Autodesk Inventor part; units mm, degrees
ref_plane "YZ Plane" through (0, 0, 0) normal (1, 0, 0) x (0, 1, 0)
ref_plane "XZ Plane" through (0, 0, 0) normal (0, 1, 0) x (-1, 0, 0)
ref_plane "XY Plane" through (0, 0, 0) normal (0, 0, 1) x (1, 0, 0)
sketch "スケッチ1" plane through (0, 0, 0) normal (0, 0, 1) x (1, 0, 0)
  circle A0 centre (0, 5.8) radius 2.6
  circle A1 centre (0, 13.4) radius 2.6
  line L0 (-3.8, 0) -> (3.8, 0)
  line L1 (3.8, 0) -> (3.8, 17.6)
  line L2 (3.8, 17.6) -> (-3.8, 17.6)
  line L3 (-3.8, 17.6) -> (-3.8, 0)
  line L4 (-11.5586, 9.6) -> (11.5586, 9.6) construction
  point P0 (0, 0)
  point P1 (0, 0)
  point P2 (0, 9.6)
  dimension "LED_DIA" = 5.2
  dimension "d1" = 7.6
  dimension "LED_PITCH" = 7.6
  dimension "TOP_MARGIN" = 4.2
  dimension "BOTTOM_MARGIN" = 5.8
extrude "スペーサ" add sketch "スケッチ1" along normal blind 5
sketch "スケッチ2" plane through (0, 0, 0) normal (0, 0, -1) x (-1, 0, 0)
  line L0 (3.8, 17.6) -> (3.8, 0)
  line L1 (-3.8, 0) -> (-3.8, 17.6)
  line L2 (3.8, 0) -> (-3.8, 0)
  line L3 (-3.8, 0) -> (-3.8, 2)
  line L4 (-3.8, 2) -> (3.8, 2)
  line L5 (3.8, 2) -> (3.8, 0)
  line L6 (3.8, 10.2) -> (-3.8, 10.2)
  line L7 (-3.8, 10.2) -> (-3.8, 9)
  line L8 (-3.8, 9) -> (3.8, 9)
  line L9 (3.8, 9) -> (3.8, 10.2)
  circle A0 centre (0, 5.8) radius 2.9 construction
  circle A1 centre (0, 13.4) radius 2.9 construction
  circle A2 centre (0, 5.8) radius 2.6 construction
  circle A3 centre (0, 13.4) radius 2.6 construction
  line L10 (6.2058, 13.4) -> (-6.2058, 13.4) construction
  line L11 (-6.2058, 5.8) -> (6.2058, 5.8) construction
  line L12 (6.2058, 9.6) -> (-6.2058, 9.6) construction
  point P0 (0, 0)
  point P1 (3.8, 9.6)
  point P2 (-3.8, 9)
  point P3 (3.8, 9)
  point P4 (3.8, 10.2)
  point P5 (-3.8, 10.2)
  dimension "d8" = 5.8
  dimension "d9" = 2
  dimension "d10" = 1.2
extrude "押し出し2" add sketch "スケッチ2" along normal blind 3 contours L0 L2 L1 L4
extrude "押し出し5" add sketch "スケッチ2" along normal blind 2 contours L0 L8 L1 L6
chamfer "面取り1" distance 0.6 angle 45 1 edges at (-2.6, 13.4, 5)
sketch "スケッチ4" plane through (-3.8, 0, 5) normal (0, -1, 0) x (1, 0, 0)
  line L0 (4.55, -5) -> (3.05, -5)
  line L1 (3.05, -5) -> (2.3, -3.701)
  line L2 (2.3, -3.701) -> (3.05, -2.4019)
  line L3 (3.05, -2.4019) -> (4.55, -2.4019)
  line L4 (4.55, -2.4019) -> (5.3, -3.701)
  line L5 (5.3, -3.701) -> (4.55, -5)
  line L6 (0, 0) -> (7.6, 0)
  point P0 (3.8, -5)
  point P1 (3.8, -3.701)
  dimension "d19" = 3
extrude "足" add sketch "スケッチ4" along normal blind 3
sketch "スケッチ5" plane through (0, 0, 5) normal (0, 0, 1) x (1, 0, 0)
  line L0 (-0.1, 5.8) -> (0.1, 5.8)
  line L1 (0.1, 5.8) -> (0.1, 17.6)
  line L2 (0.1, 17.6) -> (-0.1, 17.6)
  line L3 (-0.1, 17.6) -> (-0.1, 5.8)
  line L4 (-3.8, 0) -> (3.8, 0)
  line L5 (3.8, 17.6) -> (-3.8, 17.6)
  point P0 (0, 0)
  point P1 (0, 5.8)
  point P2 (0, 0)
  dimension "d24" = 0.2
extrude "押し出し6" cut sketch "スケッチ5" against normal blind 0.2
properties part number "LED-Spacer1"
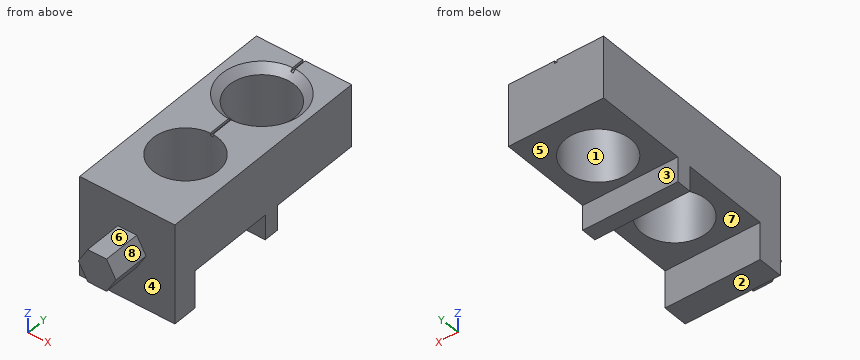
CAD build for the part. Positions are in the model's coordinates, mm. Face numbers are marked on the shaded views. A direction names the side the tool comes from. Coordinates: 2 decimals unless noted, no trailing zeros. Order: outer loops, then holes, each group sorted by start corner. A loop starts at its lowest first (then second) coordinate and runs counter-clockwise, first axis right, second up.
(1) Mould opens along Y. For the marked faces 1, 2 and 3 say: released by +Y, released by -Y, zero draft, split by the parting line, or undercut.
Solution:
face 1: undercut
face 2: zero draft
face 3: released by +Y
(2) Pin check, flat tips, straight feed: pin 1 Ø0.6 at (x, z) = (-1, -1) entering from +Y; pin 2 Ø1 at (x, z) = (-0.5, -1) entering from -Y; pin 3 Ø1.6 at (x, y) = (0, -1) entering from -Z; pin 4 Ø4 at (x, y) = (0, 13.4) entering from +Z. Stop position of each tip, or through.
Solution:
pin 1: stops at y = 10.2
pin 2: stops at y = 0
pin 3: stops at z = 0
pin 4: passes through
(3) Saw through at D-D, the plane y = -1.25. Write the cut outline in (x, z), and give its area (3 significant figures).
Solution:
outline: (-1.5, 1.3) - (-0.75, 0) - (0.75, 0) - (1.5, 1.3) - (0.75, 2.6) - (-0.75, 2.6) - close
area: 5.85 mm2
(4) Which spindle directions (+Z, -Z, +X, -X, +Y, -Y) get a long thin tool onto all of the face, cutting with end or side? Do the marked faces 4, 5, 6, 7 and 8. Say none if no direction does.
Solution:
face 4: -Y
face 5: -Z, +X, -X, +Y
face 6: +Z, +X, -X, -Y
face 7: -Z, +X, -X
face 8: +Z, +X, -Y
(5) Saw through at C-C, the plane z = 3. Write the cut outline in (x, y).
Solution:
outline: (-3.8, 0) - (3.8, 0) - (3.8, 17.6) - (-3.8, 17.6) - close; hole circle Ø5.2 at (0, 5.8); hole circle Ø5.2 at (0, 13.4)
(6) Saw through at B-B, the plane z = -1. Write the cut outline in (x, y).
Solution:
outline: (-3.8, 0) - (3.8, 0) - (3.8, 2) - (-3.8, 2) - close; (-3.8, 9) - (3.8, 9) - (3.8, 10.2) - (-3.8, 10.2) - close
(7) Saw through at A-A, the plane y = 5.8. Write the cut outline in (x, z), and give its area (3 significant figures).
Solution:
outline: (-3.8, 0) - (-2.6, 0) - (-2.6, 5) - (-3.8, 5) - close; (2.6, 0) - (3.8, 0) - (3.8, 5) - (2.6, 5) - close
area: 12.0 mm2
(8) Drill centre lines: L1, parallel to Y at x = 0, z = 2.8; L2, parallel to Y at x = 0, z = 0.9; L3, parallel to Y at x = 1.75, z = -1.25. Where is each one in solid material? Low to high.
Solution:
L1: y = 0 to 3.2, 8.4 to 10.8, 16 to 17.6
L2: y = -3 to 3.2, 8.4 to 10.8, 16 to 17.6
L3: y = 0 to 2, 9 to 10.2
